Could you check a few things on this model? Use its own coordinates, in mm. A direction names the side the tool comes from. Give positions to 0.01 mm unless a question says otherwise; leave off trailing zeros. Loops run counter-clockwise (first coordinate to the right, second up) from the corner with the lowest first, then second, coordinate; pieces in that order, holes last. Notation, with made-up numbers: (-9.5, 66) - (35.5, 66) arc R16 cw to (35.5, 87) - close; hole circle Ø3 at (-18, 17.25). An arc over 180 degrees is marked (long way). Write each question's results on one line, items separated by ' | '. Start each with the question number.
1) On a 3-axis mill with a long thin cutter (end or side, diameter ignored), from which of +Z, -Z, +X, -X, +Y, -Y can I reach the whole of each face in a straight line? I mean faces 1 (the face through (25, 2, 80)), 2 (the face through (50, 2, 63)). Say none if no direction works.
2) I want a section at C-C, the plane x = 25. Write out the boundary of the cut face in (y, z) (3 decimals).
3) I want a section at B-B, the plane z = 65. Write out the boundary of the cut face in (x, y) (3 decimals).
4) If I drill on probe 1 along X at (y, z) = (0.5, 58.5); probe 2 along X at (y, z) = (2.15, 25); probe 3 along Z at (x, y) = (21.5, 2.55), over which ranges is the centre line in solid material (lowest first)? Write a range as [from, to].
5) I'm going to push a flat-ended pin straight in: pin 1 (6 mm diameter, centred on x = 35, z = 73, fed in from +Y). Where does the tip first touch, or does it pass through?
6) If we mould it in two halves opening along Z, with no side actions, what happens to faces 3 (the face through (22.067, 1.565, 21.175)), 4 (the face through (25.55, 1.565, 0.006)), 5 (the face through (25, 0, 49))? For each: +Z half, -Z half, draft (parallel to the pull), parting line (faces both ways), or undercut.
7) I want a section at D-D, the plane z = 10. Write out the boundary of the cut face in (x, y) (3 decimals).
8) I want a section at A-A, the plane y = 0.65. Write out the boundary of the cut face in (x, z), and give its area (3 significant figures).
from build123d import *

# Parameters (mm, degrees)
SKETCH1_R           = 4.82
SKETCH1_W           = 30
SKETCH1_H           = 30
BOSS_EXTRUDE1_DEPTH = 3.175


with BuildPart() as part:
    # Sketch1 → Boss-Extrude1 (new body)
    with BuildSketch(Plane(origin=(0, 0, 0), x_dir=(1, 0, 0), z_dir=(0, 1, 0))):
        with BuildLine():
            ThreePointArc((50, -25), (25, 0), (0, -25))
            Line((0, -25), (0, -100))
            Line((0, -100), (50, -100))
            Line((50, -100), (50, -25))
        make_face()
        with Locations(Location((25, -25, 0), (0, 0, 270))):
            Circle(SKETCH1_R, mode=Mode.SUBTRACT)
        with Locations((25, -65)):
            Rectangle(SKETCH1_W, SKETCH1_H, mode=Mode.SUBTRACT)
    extrude(amount=BOSS_EXTRUDE1_DEPTH)


solid = part.part
Answers:
1) face 1: +Y, -Y | face 2: +Z, -Z, +X, +Y, -Y
2) outline: (0, 0) - (3.175, 0) - (3.175, 20.18) - (0, 20.18) - close; (0, 29.82) - (3.175, 29.82) - (3.175, 50) - (0, 50) - close; (0, 80) - (3.175, 80) - (3.175, 100) - (0, 100) - close
3) outline: (0, 0) - (10, 0) - (10, 3.175) - (0, 3.175) - close; (40, 0) - (50, 0) - (50, 3.175) - (40, 3.175) - close
4) probe 1: x = [0, 10], [40, 50] | probe 2: x = [0, 20.18], [29.82, 50] | probe 3: z = [0.25, 21.69], [28.31, 50], [80, 100]
5) pin 1: passes through
6) face 3: undercut | face 4: -Z half | face 5: draft
7) outline: (5, 0) - (45, 0) - (45, 3.175) - (5, 3.175) - close
8) outline: (0, 25) arc R25 ccw to (50, 25) - (50, 100) - (0, 100) - close; hole (10, 50) - (40, 50) - (40, 80) - (10, 80) - close; hole circle Ø9.64 at (25, 25) | area: 3,760 mm2
